The listing builds one solid part. Answer for the finished solid, in the listing's coordinates (mm). Round coordinates to 2 decimals unless told otherwise and drop trailing zeros. Write each loop counter-clockwise with the first axis right and the second up, starting at its lowest first coordinate (ties: lowest second). Pieces come first, ordered by that corner, then holes. Notation, with made-up numbers: (58, 77.5) - (99, 77.5) arc R31 ccw to (99, 104.5) - close; hole circle Ø3 at (-17.75, 58). An arc over 180 degrees is marked (long way). Use a Markdown table: item, result. Add a question column.
1) A cutting plane is placed at A-A (z = 2.7). Give the vertices of the cut face in (x, y).
2) A cutting plane is placed at B-B (y = -0.5). Give the vertices of the cut face in (x, z), then the cut area to 3 significant figures.
3) Find the intervals of material crossed by probe 1 along X at (y, z) = (21, 2.15), in increasing order. Write a range as from..to.
4) Each of these flat-tipped pins is pushed along its axis until it touches: P1, Ø1.8, axis at y = 25, z = 2.5, coming from the -X side; P2, Ø1, axis at x = 36.5, z = 1, coming from the +Y side; P3, Ø1.8, axis at x = 36.5, z = 1.5, coming from the -Y side. Where does it stop, or does it pass through?
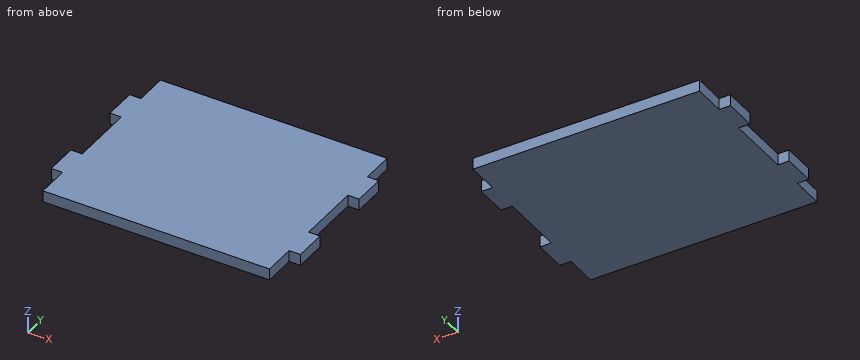
```python
from build123d import *

# Parameters (mm, degrees)
F0_W     = 70
F0_H     = 60
F1_DEPTH = 3.5
F2_W     = 10
F2_H     = 3.5
F3_DEPTH = 3.5
F4_W     = 10
F4_H     = 3.5
F5_DEPTH = 3.5


with BuildPart() as f1:
    # F0 (on Top) → F1 (new body)
    with BuildSketch(Plane.XY):
        Rectangle(F0_W, F0_H)
    extrude(amount=F1_DEPTH)

    # F2 (on face) → F3 (join)
    with BuildSketch(Plane.YZ.offset(35)):
        with Locations((-15, 1.75)):
            Rectangle(F2_W, F2_H)
        with Locations((15, 1.75)):
            Rectangle(F2_W, F2_H)
    extrude(amount=F3_DEPTH)

    # F4 (on face) → F5 (join)
    with BuildSketch(Plane(origin=(-35, 0, 0), x_dir=(0, -1, 0), z_dir=(-1, 0, 0))):
        with Locations((-15, 1.75)):
            Rectangle(F4_W, F4_H)
        with Locations((15, 1.75)):
            Rectangle(F4_W, F4_H)
    extrude(amount=F5_DEPTH)


solid = f1.part
```
Entries:
| question | item | result |
|---|---|---|
| 1 | outline | (-38.5, -20) - (-35, -20) - (-35, -30) - (35, -30) - (35, -20) - (38.5, -20) - (38.5, -10) - (35, -10) - (35, 10) - (38.5, 10) - (38.5, 20) - (35, 20) - (35, 30) - (-35, 30) - (-35, 20) - (-38.5, 20) - (-38.5, 10) - (-35, 10) - (-35, -10) - (-38.5, -10) - close |
| 2 | outline | (-35, 0) - (35, 0) - (35, 3.5) - (-35, 3.5) - close |
| 2 | area | 245 mm² |
| 3 | probe 1 | x = -35..35 |
| 4 | P1 | stops at x = -35 |
| 4 | P2 | stops at y = 20 |
| 4 | P3 | stops at y = -20 |
